```python
from build123d import *

# Parameters (mm, degrees)
SKETCH1_R           = 2.1
SKETCH1_R_2         = 2.5
SKETCH1_R_3         = 5
BOSS_EXTRUDE1_DEPTH = 1.5


with BuildPart() as part:
    # Sketch1 → Boss-Extrude1 (new body, symmetric)
    with BuildSketch(Plane.XY):
        with BuildLine():
            Line((107, -145), (107, -110.895624471))
            ThreePointArc((107, -110.895624471), (105.553363517, -102.514749396), (101.380874638, -95.103800692))
            Line((101.380874638, -95.103800692), (46.619125362, -27.896199308))
            ThreePointArc((46.619125362, -27.896199308), (42.446636483, -20.485250604), (41, -12.104375529))
            Line((41, -12.104375529), (41, 154))
            ThreePointArc((41, 154), (39.535533906, 157.535533906), (36, 159))
            Line((36, 159), (-36, 159))
            ThreePointArc((-36, 159), (-39.535533906, 157.535533906), (-41, 154))
            Line((-41, 154), (-41, -61.522167809))
            ThreePointArc((-41, -61.522167809), (-39.376465331, -70.384496434), (-34.716730508, -78.095761236))
            Line((-34.716730508, -78.095761236), (10.716730508, -129.404238764))
            ThreePointArc((10.716730508, -129.404238764), (15.198642313, -136.659946441), (16.980869565, -145))
            ThreePointArc((16.980869565, -145), (18.445335659, -148.535533906), (21.980869565, -150))
            Line((21.980869565, -150), (102, -150))
            ThreePointArc((102, -150), (105.535533906, -148.535533906), (107, -145))
        make_face()
        with Locations((96, -107)):
            Circle(SKETCH1_R, mode=Mode.SUBTRACT)
        with Locations((96, -131)):
            Circle(SKETCH1_R, mode=Mode.SUBTRACT)
        with Locations((78, -107)):
            Circle(SKETCH1_R, mode=Mode.SUBTRACT)
        with Locations((78, -131)):
            Circle(SKETCH1_R, mode=Mode.SUBTRACT)
        with Locations((46, -107)):
            Circle(SKETCH1_R, mode=Mode.SUBTRACT)
        with Locations((46, -131)):
            Circle(SKETCH1_R, mode=Mode.SUBTRACT)
        with Locations((28, -107)):
            Circle(SKETCH1_R, mode=Mode.SUBTRACT)
        with Locations((28, -131)):
            Circle(SKETCH1_R, mode=Mode.SUBTRACT)
        with Locations((-6.5, 81)):
            Circle(SKETCH1_R_2, mode=Mode.SUBTRACT)
        with Locations((-6.5, 45)):
            Circle(SKETCH1_R_2, mode=Mode.SUBTRACT)
        with Locations((-6.5, 63)):
            Circle(SKETCH1_R_3, mode=Mode.SUBTRACT)
        with Locations((51, -143)):
            Circle(SKETCH1_R, mode=Mode.SUBTRACT)
        with Locations((73, -143)):
            Circle(SKETCH1_R, mode=Mode.SUBTRACT)
        with Locations((0, 126)):
            Circle(SKETCH1_R, mode=Mode.SUBTRACT)
        Circle(SKETCH1_R, mode=Mode.SUBTRACT)
        with Locations((-32.666666667, 144)):
            Circle(SKETCH1_R, mode=Mode.SUBTRACT)
        with Locations((-17.333333333, 124)):
            Circle(SKETCH1_R, mode=Mode.SUBTRACT)
        with Locations((-17.333333333, -31)):
            Circle(SKETCH1_R, mode=Mode.SUBTRACT)
        with Locations((-32.666666667, -51)):
            Circle(SKETCH1_R, mode=Mode.SUBTRACT)
    extrude(amount=BOSS_EXTRUDE1_DEPTH, both=True)


solid = part.part
```
Part model, mm, in its own coordinate system. Round coordinates to 2 decimals unless told otherwise and drop trailing zeros. Write each loop counter-clockwise with the first axis right and the second up, starting at its lowest first coordinate (ties: lowest second). Pieces come first, ordered by that corner, then holes.
Item 1: Cut at D-D, the plane x = 58.5. Give the cut face in (y, z).
Results:
outline: (-150, -1.5) - (-42.48, -1.5) - (-42.48, 1.5) - (-150, 1.5) - close
Item 2: Two-plate mould, pull along Y, no slides. Class faces 1 (the cylindrical face through (-3.812, 67.216, -0.021)), 2 (the flat face through (16, 7, -1.5)), 3 (the cylindrical face through (42.487, -20.598, 0.021)): +Y half, -Y half, draft (parallel to the pull), parting line (faces both ways), or undercut.
Results:
face 1: undercut
face 2: draft
face 3: +Y half
Item 3: Drop a flat-ended pin along its axis: pin 1 Ø0.9 at (y, z) = (106.5, 0) entering from +X. Give the stop position or say it passes through.
Results:
pin 1: stops at x = 41
Item 4: Probe L1, parallel to X at y = -131, z = 0.15; L2, parallel to Y at x = 28, z = 0.7; L3, parallel to Y at x = 96, z = -0.1. List the from-to ranges inside material, lowest first.
Results:
L1: x = 12.02 to 25.9, 30.1 to 43.9, 48.1 to 75.9, 80.1 to 93.9, 98.1 to 107
L2: y = -150 to -133.1, -128.9 to -109.1, -104.9 to 159
L3: y = -150 to -133.1, -128.9 to -109.1, -104.9 to -88.5
Item 5: Cut at A-A, the plane y = 63. Give the cut face in (x, z).
Results:
outline: (-41, -1.5) - (-11.5, -1.5) - (-11.5, 1.5) - (-41, 1.5) - close; (-1.5, -1.5) - (41, -1.5) - (41, 1.5) - (-1.5, 1.5) - close
Item 6: Cut at B-B, the plane z = -0.7. Count the separate pieces of the cut face and the enclosed holes in it, plus the area to 3 significant figures.
Results:
separate pieces: 1
enclosed holes: 19
area: 28,100 mm2
Item 7: Cut at C-C, the plane y = 94.5. Give the cut face in (x, z), plus the area to 3 significant figures.
Results:
outline: (-41, -1.5) - (41, -1.5) - (41, 1.5) - (-41, 1.5) - close
area: 246 mm2
